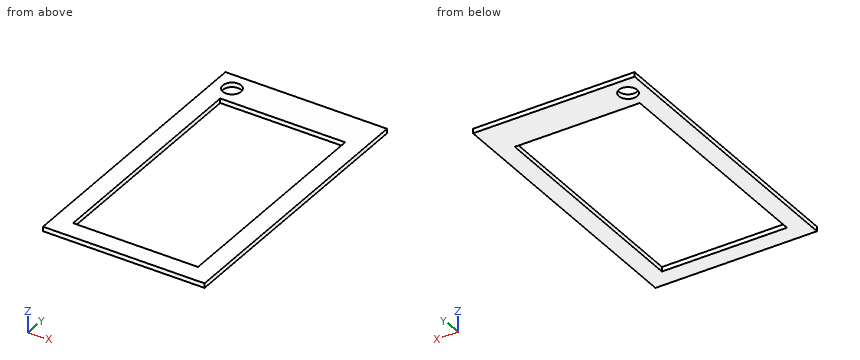
from build123d import *

# Parameters (mm, degrees)
F0_R     = 3.175
F1_DEPTH = 1.5875


with BuildPart() as f1:
    # F0 (on Top) → F1 (new body)
    with BuildSketch(Plane.XY):
        Polygon((21.693888, -42.8625), (21.693888, 0), (21.693888, 36.5125), (0, 36.5125), (-21.693888, 36.5125), (-21.693888, 0), (-21.693888, -42.8625), (0, -42.8625), align=None)
        Polygon((-28.043888, -49.2125), (28.043888, -49.2125), (28.043888, 0), (28.043888, 35.28102), (28.043888, 49.2125), (0, 49.2125), (-28.043888, 49.2125), (-28.043888, 35.28102), align=None)
        Polygon((21.693888, 36.5125), (21.693888, 0), (21.693888, -42.8625), (0, -42.8625), (-21.693888, -42.8625), (-21.693888, 0), (-21.693888, 36.5125), (0, 36.5125), align=None, mode=Mode.SUBTRACT)
        with Locations((-21.693888, 42.8625)):
            Circle(F0_R, mode=Mode.SUBTRACT)
    extrude(amount=F1_DEPTH)


solid = f1.part
For this review, take the finished solid that the model builds, in its own axes (mm). Give positions to 0.01 mm unless a question says otherwise; leave off trailing zeros. Order: outer loops, then holes, each group sorted by start corner. A loop starts at its lowest first (then second) coordinate and runs counter-clockwise, first axis right, second up. Notation, with made-up numbers: (-17.5, -12) -> (9.5, -12) arc R23 ccw to (9.5, 2) -> close; hole circle Ø11 at (-23.75, 20.5). An arc over 180 degrees is marked (long way). Write item = value, one per line.
1) We need section A-A, the plane y = -22.5. Give the boundary of the cut face in (x, z), and give its area (3 significant figures).
Findings:
outline = (-28.04, 0) -> (-21.69, 0) -> (-21.69, 1.59) -> (-28.04, 1.59) -> close; (21.69, 0) -> (28.04, 0) -> (28.04, 1.59) -> (21.69, 1.59) -> close
area = 20.2 mm^2
2) We need section C-C, the plane z = 0.7. Count the separate pieces of the cut face and the enclosed holes in it, and give its area (3 significant figures).
Findings:
separate_pieces = 1
enclosed_holes = 2
area = 2,040 mm^2
3) To check wall thickness, follow L1, parallel to X at y = 14.5, z = 0.3; L2, parallel to Y at x = -3, z = 1.5; L3, parallel to X at y = 43, z = 0.3. State the ranges of each line that lie inside material, in increasing order. Write a range as from..to.
Findings:
L1 = -28.04..-21.69, 21.69..28.04
L2 = -49.21..-42.86, 36.51..49.21
L3 = -28.04..-24.87, -18.52..28.04
4) Insertion check: pin 1 (10 mm diameter, centred on x = 12.5, y = 19, fed in from +Z); pin 2 (1 mm diameter, centred on x = 21.5, y = -5, fed in from +Z). Each pin has a flat end and moves straight along its axis. Give the tip position at first contact, or say it passes through.
Findings:
pin_1 = through
pin_2 = 1.59
5) We need section B-B, the plane x = -9. Give the boundary of the cut face in (y, z).
Findings:
outline = (-49.21, 0) -> (-42.86, 0) -> (-42.86, 1.59) -> (-49.21, 1.59) -> close; (36.51, 0) -> (49.21, 0) -> (49.21, 1.59) -> (36.51, 1.59) -> close
